from build123d import *

# Parameters (mm, degrees)
F0_R     = 35
F0_R_2   = 5.5
F0_R_3   = 50
F0_R_4   = 29
F0_R_5   = 21
F1_DEPTH = 55
F2_DEPTH = 10
F4_DEPTH = 5
F5_R     = 8
F6_DEPTH = 25
F7_R     = 8
F8_DEPTH = 25


# Not quite as in the source:
# - ends of sketch curves that miss each other by under 0.0002 mm in the source are joined


with BuildPart() as f1:
    # F0 (on Top) → F1 (new body)
    with BuildSketch(Plane.XY):
        with BuildLine():
            ThreePointArc((-265, -55), (-261.4644660941, -63.5355339059), (-270, -60))
            Line((-270, -60), (-320, -60))
            Line((-320, -60), (-320, -90))
            ThreePointArc((-320, -90), (-319.427901562, -94.7493832125), (-317.7443359101, -99.2270549532))
            Line((-317.7443359101, -99.2270549532), (-252.744336, -224.227055))
            ThreePointArc((-252.744336, -224.227055), (-245.3792798627, -232.0959220147), (-235, -235))
            Line((-235, -235), (235, -235))
            ThreePointArc((235, -235), (245.3792798627, -232.0959220147), (252.7443359101, -224.2270549532))
            Line((252.7443359101, -224.2270549532), (317.744336, -99.227055))
            ThreePointArc((317.744336, -99.227055), (319.427901562, -94.7493832125), (320, -90))
            Line((320, -90), (320, -60))
            Line((320, -60), (270, -60))
            ThreePointArc((270, -60), (261.4644660941, -63.5355339059), (265, -55))
            Line((265, -55), (265, 55))
            ThreePointArc((265, 55), (261.4644660941, 63.5355339059), (270, 60))
            Line((270, 60), (320, 60))
            Line((320, 60), (320, 90))
            ThreePointArc((320, 90), (319.427901562, 94.7493832125), (317.7443359101, 99.2270549532))
            Line((317.7443359101, 99.2270549532), (252.744336, 224.227055))
            ThreePointArc((252.744336, 224.227055), (245.3792798627, 232.0959220147), (235, 235))
            Line((235, 235), (-235, 235))
            ThreePointArc((-235, 235), (-245.3792798627, 232.0959220147), (-252.7443359101, 224.2270549532))
            Line((-252.7443359101, 224.2270549532), (-317.744336, 99.227055))
            ThreePointArc((-317.744336, 99.227055), (-319.427901562, 94.7493832125), (-320, 90))
            Line((-320, 90), (-320, 60))
            Line((-320, 60), (-270, 60))
            ThreePointArc((-270, 60), (-261.4644660941, 63.5355339059), (-265, 55))
            Line((-265, 55), (-265, -55))
        make_face()
        with Locations((-195, -195)):
            Circle(F0_R, mode=Mode.SUBTRACT)
        with Locations((-150, -150)):
            Circle(F0_R_2, mode=Mode.SUBTRACT)
        with Locations((150, -150)):
            Circle(F0_R_2, mode=Mode.SUBTRACT)
        with Locations((195, -194.81006)):
            Circle(F0_R, mode=Mode.SUBTRACT)
        with Locations((0, -0.1899)):
            Circle(F0_R_3, mode=Mode.SUBTRACT)
        with Locations((-195, 195)):
            Circle(F0_R, mode=Mode.SUBTRACT)
        with Locations((-150, 150)):
            Circle(F0_R_2, mode=Mode.SUBTRACT)
        with Locations((150, 150)):
            Circle(F0_R_2, mode=Mode.SUBTRACT)
        with Locations((195, 194.810059)):
            Circle(F0_R, mode=Mode.SUBTRACT)
        with Locations((0, -0.1899)):
            Circle(F0_R_3)
        with Locations((0, 4e-05)):
            Circle(F0_R_4, mode=Mode.SUBTRACT)
        with Locations((-195, 195)):
            Circle(F0_R)
        with Locations((-195, 195)):
            Circle(F0_R_5, mode=Mode.SUBTRACT)
        with Locations((195, 194.810059)):
            Circle(F0_R)
        with Locations((195, 194.810059)):
            Circle(F0_R_5, mode=Mode.SUBTRACT)
        with Locations((-195, -195)):
            Circle(F0_R)
        with Locations((-195, -195)):
            Circle(F0_R_5, mode=Mode.SUBTRACT)
        with Locations((195, -194.81006)):
            Circle(F0_R)
        with Locations((195, -194.81006)):
            Circle(F0_R_5, mode=Mode.SUBTRACT)
    extrude(amount=F1_DEPTH)

    # F0 (on Top) → F2 (cut)
    with BuildSketch(Plane.XY):
        with Locations((195, 194.810059)):
            Circle(F0_R)
        with Locations((195, 194.810059)):
            Circle(F0_R_5, mode=Mode.SUBTRACT)
        with Locations((-195, 195)):
            Circle(F0_R)
        with Locations((-195, 195)):
            Circle(F0_R_5, mode=Mode.SUBTRACT)
        with Locations((0, -0.1899)):
            Circle(F0_R_3)
        with Locations((0, 4e-05)):
            Circle(F0_R_4, mode=Mode.SUBTRACT)
        with Locations((-195, -195)):
            Circle(F0_R)
        with Locations((-195, -195)):
            Circle(F0_R_5, mode=Mode.SUBTRACT)
        with Locations((195, -194.81006)):
            Circle(F0_R)
        with Locations((195, -194.81006)):
            Circle(F0_R_5, mode=Mode.SUBTRACT)
    extrude(amount=F2_DEPTH, mode=Mode.SUBTRACT)

    # F3 (on face) → F4 (cut)
    with BuildSketch(Plane.XY.offset(55)):
        with BuildLine():
            Line((270, 60), (320, 60))
            Line((320, 60), (320, 90))
            ThreePointArc((320, 90), (319.427901562, 94.7493832125), (317.7443359101, 99.2270549532))
            Line((317.7443359101, 99.2270549532), (252.744336, 224.227055))
            ThreePointArc((252.744336, 224.227055), (251.4939773544, 226.311441724), (250, 228.2287566232))
            Line((250, 228.2287566232), (250, -228.2287565553))
            ThreePointArc((250, -228.2287565553), (251.4939773092, -226.3114416643), (252.7443359101, -224.2270549532))
            Line((252.7443359101, -224.2270549532), (317.744336, -99.227055))
            ThreePointArc((317.744336, -99.227055), (319.4279015605, -94.7493832184), (320, -90))
            Line((320, -90), (320, -60))
            Line((320, -60), (270, -60))
            ThreePointArc((270, -60), (261.4644660941, -63.5355339059), (265, -55))
            Line((265, -55), (265, 55))
            ThreePointArc((265, 55), (261.4644660941, 63.5355339059), (270, 60))
        make_face()
        with BuildLine():
            Line((-250, -228.2287566232), (-250, 228.2287565553))
            ThreePointArc((-250, 228.2287565553), (-251.4939773092, 226.3114416643), (-252.7443359101, 224.2270549532))
            Line((-252.7443359101, 224.2270549532), (-317.744336, 99.227055))
            ThreePointArc((-317.744336, 99.227055), (-319.4279015605, 94.7493832184), (-320, 90))
            Line((-320, 90), (-320, 60))
            Line((-320, 60), (-270, 60))
            ThreePointArc((-270, 60), (-261.4644660941, 63.5355339059), (-265, 55))
            Line((-265, 55), (-265, -55))
            ThreePointArc((-265, -55), (-261.4644660941, -63.5355339059), (-270, -60))
            Line((-270, -60), (-320, -60))
            Line((-320, -60), (-320, -90))
            ThreePointArc((-320, -90), (-319.427901562, -94.7493832125), (-317.7443359101, -99.2270549532))
            Line((-317.7443359101, -99.2270549532), (-252.744336, -224.227055))
            ThreePointArc((-252.744336, -224.227055), (-251.4939773544, -226.311441724), (-250, -228.2287566232))
        make_face()
    extrude(amount=-F4_DEPTH, mode=Mode.SUBTRACT)

    # F5 (on face) → F6 (cut)
    with BuildSketch(Plane.YZ.offset(265)):
        with Locations((30, 25)):
            Circle(F5_R)
        with Locations((-30, 25)):
            Circle(F5_R)
    extrude(amount=-F6_DEPTH, mode=Mode.SUBTRACT)

    # F7 (on face) → F8 (cut)
    with BuildSketch(Plane(origin=(-265, 0, 0), x_dir=(0, -1, 0), z_dir=(-1, 0, 0))):
        with Locations((-30, 25)):
            Circle(F7_R)
        with Locations((30, 25)):
            Circle(F7_R)
    extrude(amount=-F8_DEPTH, mode=Mode.SUBTRACT)


solid = f1.part
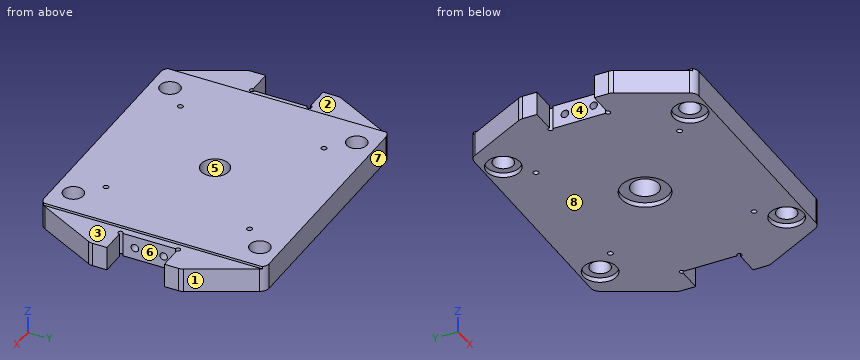
Build history of the part. All positions in model axes, mm. Face numbers are marked on the shaded views. A direction names the side the tool comes from. Give positions to 0.01 mm unless a question says otherwise; leave off trailing zeros. Loops run counter-clockwise (first coordinate to the right, second up) from the corner with the lowest first, then second, coordinate; pieces in that order, holes last. Notation, with made-up numbers: (11.25, 22.5) -> (43.25, 22.5) arc R22 cw to (43.25, 45.5) -> close; hole circle Ø4 at (-14.75, -4.75). An arc over 180 degrees is marked (long way). Answer in a Markdown table with one row per item.
Item 1: Slice it at C-C on y = -127. Write the cut outline in (x, z), plus the area to 3 significant figures.
Findings below:
| item | result |
|---|---|
| outline | (-303.3, 0) -> (303.3, 0) -> (303.3, 50) -> (250, 50) -> (250, 55) -> (-250, 55) -> (-250, 50) -> (-303.3, 50) -> close |
| area | 32,800 mm² |
Item 2: Slice it at A-A on x = 0. Write the cut outline in (y, z), plus the area to 3 significant figures.
Findings below:
| item | result |
|---|---|
| outline | (-235, 0) -> (-50.19, 0) -> (-50.19, 10) -> (-29, 10) -> (-29, 55) -> (-235, 55) -> close; (29, 10) -> (49.81, 10) -> (49.81, 0) -> (235, 0) -> (235, 55) -> (29, 55) -> close |
| area | 22,200 mm² |
Item 3: Probe line 1 along Y through (x, z) = (-150, 33.5); line 2 along Y through (x, z) = (-195, 6.25); line 3 along X through (y, z) = (197.5, 12.5). List the from-to ranges inside material, lowest first. Write a range as [from, to].
Findings below:
| item | result |
|---|---|
| line 1 | y = [-235, -155.5], [-144.5, 144.5], [155.5, 235] |
| line 2 | y = [-235, -230], [-160, 160], [230, 235] |
| line 3 | x = [-266.64, -215.85], [-174.15, 174.17], [215.83, 266.64] |
Item 4: Slice it at D-D on z = 25. Give the number of separate pieces and of enclosed holes in the cut face, plus the area to 3 significant figures.
Findings below:
| item | result |
|---|---|
| separate pieces | 1 |
| enclosed holes | 9 |
| area | 257,000 mm² |
Item 5: Flat gauge pins, fed straight in: P1, Ø5.5, axis at y = -20, z = 53, coming from the -X side; P2, Ø8, axis at y = -27.5, z = 27, coming from the -X side; P3, Ø4, axis at y = 183, z = 11, coming from the +X side; P4, Ø10, axis at x = 150, y = -150, coming from the +Z side. Where does each tip first touch, or does it go through?
Findings below:
| item | result |
|---|---|
| P1 | stops at x = -250 |
| P2 | stops at x = -240 |
| P3 | stops at x = 275.22 |
| P4 | passes through |
Item 6: Slice it at B-B on x = 195. Write the cut outline in (y, z).
Findings below:
| item | result |
|---|---|
| outline | (-235, 0) -> (-229.81, 0) -> (-229.81, 10) -> (-215.81, 10) -> (-215.81, 55) -> (-235, 55) -> close; (-173.81, 10) -> (-159.81, 10) -> (-159.81, 0) -> (159.81, 0) -> (159.81, 10) -> (173.81, 10) -> (173.81, 55) -> (-173.81, 55) -> close; (215.81, 10) -> (229.81, 10) -> (229.81, 0) -> (235, 0) -> (235, 55) -> (215.81, 55) -> close |
Item 7: Tool access for the marked faces 1, 2, 3, 4 and 5: list every direction of +Z, -Z, +X, -X, +Y, -Y with a clear straight run to the whole face (end or side of a thin tool).
Findings below:
| item | result |
|---|---|
| face 1 | +Z, -Z, +X, +Y |
| face 2 | +Z, -X, +Y, -Y |
| face 3 | +Z, +X, +Y, -Y |
| face 4 | +Z, -Z, -X |
| face 5 | +Z, -Z |
Item 8: Mould opens along Y. For the marked faces 6, 7 and 8 say: pulls with the +Y half, pulls with the -Y half, needs draft (parallel to the pull), parting line crosses it, or undercut.
Findings below:
| item | result |
|---|---|
| face 6 | undercut |
| face 7 | pulls with the +Y half |
| face 8 | needs draft |
